```python
from build123d import *

# Parameters (mm, degrees)
F0_W     = 62.25
F0_H     = 37.5
F0_W_2   = 6.35
F0_H_2   = 6.35
F1_DEPTH = 1.6
F2_DEPTH = 2.5
F3_D     = 1.3
F4_D     = 3.25


with BuildPart() as f1:
    # F0 (on Top) → F1 (new body)
    with BuildSketch(Plane.XY):
        Rectangle(F0_W, F0_H)
        with Locations((2.3, -7.275)):
            Rectangle(F0_W_2, F0_H_2, mode=Mode.SUBTRACT)
        with Locations((2.3, -7.275)):
            Rectangle(F0_W_2, F0_H_2)
    extrude(amount=-F1_DEPTH)

    # F0 (on Top) → F2 (join)
    with BuildSketch(Plane.XY):
        with Locations((2.3, -7.275)):
            Rectangle(F0_W_2, F0_H_2)
    extrude(amount=F2_DEPTH)

    # F3 (through all)
    with Locations(Plane.XY):
        with Locations((-13.325, 13.75), (-10.785, 13.75), (-8.245, 13.75), (-27.375, 3.4), (-27.375, 0.86), (-27.375, -1.68), (-27.375, -4.22), (-27.375, -6.76), (-27.375, -9.3), (5.365, -13.75), (7.905, -13.75), (10.445, -13.75), (12.985, -13.75), (26.685, -5.4), (26.685, -2.86), (26.685, -0.32), (26.685, 2.22), (26.685, 4.76)):
            Hole(F3_D / 2)

    # F4 (through all)
    with Locations(Plane.XY):
        with Locations((-27.25, 14.72), (-27.25, -14.72), (27.25, -14.72), (27.25, 14.72)):
            Hole(F4_D / 2)


solid = f1.part
```
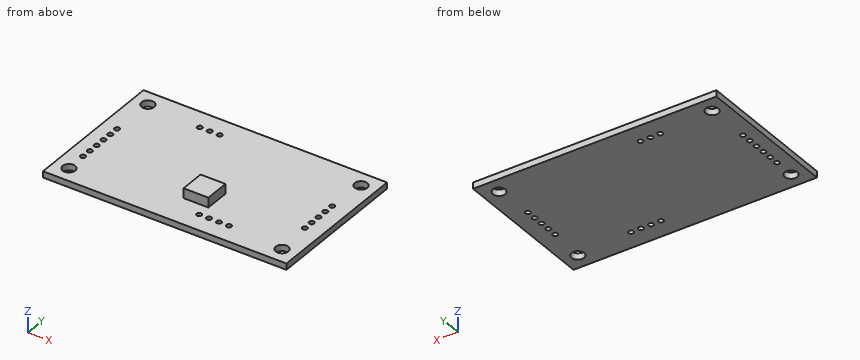
Could you check a few things on this model? Use its own coordinates, in mm. Give positions to 0.01 mm unless a question says otherwise; leave off trailing zeros. Write each loop counter-clockwise with the first axis right and the second up, starting at its lowest first coordinate (ties: lowest second). Pieces come first, ordered by that corner, then holes. Notation, with made-up numbers: (72.25, 64.25) -> (83.25, 64.25) arc R20 ccw to (83.25, 85.25) -> close; hole circle Ø7 at (12, 14.5). An arc over 180 degrees is marked (long way). Write each question's results on one line, items separated by ' | '.
1. I need wall thicknesses on L1, parallel to Z at x = 9.5, y = 15; L2, parallel to X at y = 2, z = -0.15 (3 decimals). Which ranges of each line are inside material? Lowest first, please.
Check sheet entries:
L1: z = -1.6 to 0 | L2: x = -31.125 to 26.073, 27.297 to 31.125
2. I want a section at A-A, the plane y = -13.75. Write out the boundary of the cut face in (x, z) (3 decimals).
Check sheet entries:
outline: (-31.125, -1.6) -> (-28.554, -1.6) -> (-28.554, 0) -> (-31.125, 0) -> close; (-25.946, -1.6) -> (4.715, -1.6) -> (4.715, 0) -> (-25.946, 0) -> close; (6.015, -1.6) -> (7.255, -1.6) -> (7.255, 0) -> (6.015, 0) -> close; (8.555, -1.6) -> (9.795, -1.6) -> (9.795, 0) -> (8.555, 0) -> close; (11.095, -1.6) -> (12.335, -1.6) -> (12.335, 0) -> (11.095, 0) -> close; (13.635, -1.6) -> (25.946, -1.6) -> (25.946, 0) -> (13.635, 0) -> close; (28.554, -1.6) -> (31.125, -1.6) -> (31.125, 0) -> (28.554, 0) -> close
3. I want a section at B-B, the plane z = -0.7. Count the separate pieces of the cut face and the enclosed holes in it, then the cut area to 3 significant figures.
Check sheet entries:
separate pieces: 1 | enclosed holes: 22 | area: 2,280 mm²
4. Will these pins go through, and if not, where does the flat tip stop? pin 1 Ø1.2 at (x, z) = (1.5, 1) entering from -Y; pin 2 Ø1 at (x, y) = (-10.785, 13.75) entering from +Z; pin 3 Ø2 at (x, y) = (4, -3) entering from +Z.
Check sheet entries:
pin 1: stops at y = -10.45 | pin 2: passes through | pin 3: stops at z = 0
5. I want a section at C-C, the plane x = 3. Write out the boundary of the cut face in (y, z), then the cut area to 3 significant figures.
Check sheet entries:
outline: (-18.75, -1.6) -> (18.75, -1.6) -> (18.75, 0) -> (-4.1, 0) -> (-4.1, 2.5) -> (-10.45, 2.5) -> (-10.45, 0) -> (-18.75, 0) -> close | area: 75.9 mm²
6. I want a section at D-D, the plane y = 15.5. Write out the boundary of the cut face in (x, z) (3 decimals), then the cut area to 3 significant figures.
Check sheet entries:
outline: (-31.125, -1.6) -> (-28.676, -1.6) -> (-28.676, 0) -> (-31.125, 0) -> close; (-25.824, -1.6) -> (25.824, -1.6) -> (25.824, 0) -> (-25.824, 0) -> close; (28.676, -1.6) -> (31.125, -1.6) -> (31.125, 0) -> (28.676, 0) -> close | area: 90.5 mm²
